from build123d import *

# Parameters (mm, degrees)
BOSS_EXTRUDE1_DEPTH                            = 55
SKETCH6_W                                      = 47
SKETCH6_H                                      = 10.5
CUT_EXTRUDE3_DEPTH                             = 55
CHAMFER3_SIZE                                  = 5
CHAMFER4_SIZE                                  = 5
CSK_FOR_M3_FLAT_HEAD_MACHINE_SCREW1_AT_2_COUNT = 2
CSK_FOR_M3_FLAT_HEAD_MACHINE_SCREW1_AT_2_PITCH = 13.5
CSK_FOR_M3_FLAT_HEAD_MACHINE_SCREW1_AT_3_COUNT = 2
CSK_FOR_M3_FLAT_HEAD_MACHINE_SCREW1_AT_3_PITCH = 47
CSK_FOR_M3_FLAT_HEAD_MACHINE_SCREW1_AT_4_COUNT = 2
CSK_FOR_M3_FLAT_HEAD_MACHINE_SCREW1_AT_4_PITCH = 33.5
TAP_DRILL_FOR_M3X0_5_TAP1_D                    = 2.5
FILLET1_R                                      = 0.5


# Read off the part's stored shape, not the designer's step: Body-Delete/Keep 1
with BuildPart() as part:
    # Sketch1 → Boss-Extrude1 (new body)
    with BuildSketch(Plane.XY):
        Polygon((22, -20), (25, -20), (25, 1.035533906), (27.5, 3.535533906), (30, 1.035533906), (30, 9.035533906), (25, 9.035533906), (25, 35), (22, 35), align=None)
    extrude(amount=BOSS_EXTRUDE1_DEPTH)

    # Sketch4 → Cut-Revolve1 (revolve, cut)
    with BuildSketch(Plane(origin=(0, 0, 0), x_dir=(1, 0, 0), z_dir=(0, 1, 0))):
        Polygon((27.5, -47.011533546), (30, -47.011533546), (31.5, -55.011533546), (27.5, -55.011533546), align=None)
    revolve(axis=Axis((27.5, 0, 0), (0, 0, 1)), mode=Mode.SUBTRACT)

    # Sketch6 → Cut-Extrude3 (cut)
    with BuildSketch(Plane.ZY.offset(-22)):
        Polygon((55, 6), (55, 35), (8, 35), (8, 27), align=None)
        with Locations((31.5, -14.75)):
            Rectangle(SKETCH6_W, SKETCH6_H)
    extrude(amount=-CUT_EXTRUDE3_DEPTH, mode=Mode.SUBTRACT)

    # Chamfer3
    chamfer3_edges = [part.edges().sort_by_distance(p)[0] for p in [
        (23.5, -9.5, 55),
        (23.5, -9.5, 8),
    ]]
    chamfer(chamfer3_edges, length=CHAMFER3_SIZE)

    # Chamfer4
    chamfer4_edges = [part.edges().sort_by_distance(p)[0] for p in [
        (30, 9.035533906, 24.10309301),
    ]]
    chamfer(chamfer4_edges, length=CHAMFER4_SIZE - 0.0001)  # a hair under: the kernel refuses the full size

    # Sketch8 → CSK for M3 Flat Head Machine Screw1 (revolve, cut)
    with BuildSketch(Plane(origin=(25, 31, 4), x_dir=(0, 0, -1), z_dir=(0, 1, 0))):
        Polygon((0, 0), (0, 3), (1.6, 3), (1.6, 1.55), (3.15, 0), align=None)
    csk_for_m3_flat_head_machine_screw1 = revolve(axis=Axis((31.35, 31, 4), (-1, 0, 0)), mode=Mode.SUBTRACT)

    # CSK for M3 Flat Head Machine Screw1 at 2: CSK for M3 Flat Head Machine Screw1 ×2
    with Locations(*[(0, -i * CSK_FOR_M3_FLAT_HEAD_MACHINE_SCREW1_AT_2_PITCH, 0) for i in range(1, CSK_FOR_M3_FLAT_HEAD_MACHINE_SCREW1_AT_2_COUNT)]):
        add(csk_for_m3_flat_head_machine_screw1, mode=Mode.SUBTRACT)

    # CSK for M3 Flat Head Machine Screw1 at 3: CSK for M3 Flat Head Machine Screw1 ×2
    with Locations(*[(0, -i * CSK_FOR_M3_FLAT_HEAD_MACHINE_SCREW1_AT_3_PITCH, 0) for i in range(1, CSK_FOR_M3_FLAT_HEAD_MACHINE_SCREW1_AT_3_COUNT)]):
        add(csk_for_m3_flat_head_machine_screw1, mode=Mode.SUBTRACT)

    # CSK for M3 Flat Head Machine Screw1 at 4: CSK for M3 Flat Head Machine Screw1 ×2
    with Locations(*[(0, -i * CSK_FOR_M3_FLAT_HEAD_MACHINE_SCREW1_AT_4_PITCH, 0) for i in range(1, CSK_FOR_M3_FLAT_HEAD_MACHINE_SCREW1_AT_4_COUNT)]):
        add(csk_for_m3_flat_head_machine_screw1, mode=Mode.SUBTRACT)

    # Tap Drill for M3x0.5 Tap1 (through all)
    with Locations(Plane(origin=(25, 0, 0), x_dir=(0, 0, -1), z_dir=(1, 0, 0))):
        with Locations((-41, -6.5), (-34, -6.5)):
            Hole(TAP_DRILL_FOR_M3X0_5_TAP1_D / 2)

    # Fillet1
    fillet1_edges = [part.edges().sort_by_distance(p)[0] for p in [
        (23.5, -20, 0),
        (23.5, 27, 8),
        (23.5, 35, 8),
        (23.5, -20, 8),
        (23.5, -14.5, 8),
        (23.5, -9.5, 50),
        (23.5, -9.5, 13),
        (23.5, -4.5, 55),
        (23.5, 35, 0),
    ]]
    fillet(fillet1_edges, radius=FILLET1_R)


with BuildPart() as body_2:
    # Mirror2: mirrored copy
    add(part.part.mirror(Plane(origin=(22, -20, 55), x_dir=(0, 0, 1), z_dir=(1, 0, 0))))


solid = body_2.part
Geometry: final body of the model. Coordinates: model frame, mm. A direction names the side the tool comes from. Give positions to 0.01 mm unless a question says otherwise; leave off trailing zeros. Order: outer loops, then holes, each group sorted by start corner. A loop starts at its lowest first (then second) coordinate and runs counter-clockwise, first axis right, second up. Notation, with made-up numbers: (53.25, 37) -> (108.25, 37) arc R10 cw to (108.25, 55) -> close; hole circle Ø11 at (60.5, -22.5). An arc over 180 degrees is marked (long way). Write each question's results on one line, items separated by ' | '.
1) Cut plane B-B (x = 21.25). Output: boundary loops of the cut face in (y, z).
Geometry says:
outline: (-20, 0.5) arc R0.5 ccw to (-19.5, 0) -> (34.5, 0) arc R0.5 ccw to (35, 0.5) -> (35, 7.5) arc R0.5 ccw to (34.5, 8) -> (27.32, 8) arc R0.5 cw to (26.87, 8.3) -> (6, 55) -> (-4.29, 55) arc R0.5 ccw to (-4.65, 54.85) -> (-9.35, 50.15) arc R0.5 ccw to (-9.5, 49.79) -> (-9.5, 13.21) arc R0.5 cw to (-9.65, 12.85) -> (-14.35, 8.15) arc R0.5 cw to (-14.71, 8) -> (-19.5, 8) arc R0.5 ccw to (-20, 7.5) -> close; hole circle Ø3.2 at (-16, 4); hole circle Ø2.5 at (-6.5, 34); hole circle Ø2.5 at (-6.5, 41); hole circle Ø3.2 at (-2.5, 4); hole circle Ø3.2 at (17.5, 4); hole circle Ø3.2 at (31, 4)
2) Set-up query: faces 5 (the face through (21, 31, 8)), 6 (the face through (15.267, 2.303, 25.899)), 7 (the face through (19, 16, 18)). Return all of +Z, -Z, +X, -X, +Y, -Y with unobstructed straight access to the full face (end or side cutting, diameter ignored); none if empty.
Geometry says:
face 5: +Z, +X, -X, +Y | face 6: +Z, -Z, -Y | face 7: +Z, -Z, -X, +Y
3) Cut plane C-C (y = -16). Output: boundary loops of the cut face in (x, z), and give its area (3 significant figures).
Geometry says:
outline: (19, 0) -> (22, 0) -> (22, 2.4) -> (20.55, 2.4) -> (19, 0.85) -> close; (19, 7.15) -> (20.55, 5.6) -> (22, 5.6) -> (22, 8) -> (19, 8) -> close | area: 12.0 mm²
4) First-contact query: pin 1 Ø1.5 at (x, z) = (21, 25.5) entering from -Y; pin 2 Ø21 at (y, z) = (20, 35) entering from -X; pin 3 Ø3 at (x, z) = (17, 28.5) entering from +Y; pin 4 Ø2 at (x, y) = (17, 26.5) entering from -Z. Flat tips, straight axial feed; report the tip coordinate or a pass-through.
Geometry says:
pin 1: stops at y = -9.5 | pin 2: stops at x = 19 | pin 3: stops at y = 8.54 | pin 4: passes through
5) Line query: line 1 along Y through (x, z) = (21.4, 4); line 2 along Z through (x, y) = (21.35, -16); line 3 along X through (y, z) = (26, 10). Output: solid intervals per line, ascending.
Geometry says:
line 1: y = -20 to -17.6, -14.4 to -4.1, -0.9 to 15.9, 19.1 to 29.4, 32.6 to 35 | line 2: z = 0 to 2.4, 5.6 to 8 | line 3: x = 19 to 22
6) Draft query along X for faces 1 (the face through (18.39, 2.656, 51.062)), 2 (the face through (21.265, -17.586, 4.208)), 3 (the face through (19, -5, 27)), 4 (the face through (17.767, 2.268, 25.899)). Return one class per face: released by +X, released by -X, zero draft, split by the parting line, or undercut.
Geometry says:
face 1: undercut | face 2: zero draft | face 3: released by -X | face 4: undercut
7) Cut plane A-A (z = 4). Give the number of separate pieces and of enclosed holes in the cut face, and give its area (3 significant figures).
Geometry says:
separate pieces: 5 | enclosed holes: 0 | area: 138 mm²
